Geometry: final body of the model. Coordinates: model frame, mm. Give positions to 0.01 mm unless a question says otherwise; leave off trailing zeros. Write each loop counter-clockwise with the first axis right and the second up, starting at its lowest first coordinate (ties: lowest second). Pieces come first, ordered by that corner, then holes. Notation, with made-up numbers: (71, 10.5) -> (118, 10.5) arc R11 cw to (118, 28.5) -> close; hole circle Ø3 at (35, -28.75). An arc over 180 degrees is marked (long way). Answer as a JSON object with one key per item and string values. Group by question number.
(1) Material intervals for probe 1 along X at (y, z) = (-51.5, 0.2); probe 2 along Y at (x, z) = (15.5, 0.8); probe 3 along Y at (x, z) = (-36, 0.35), sorted ascending.
(2) Section query B-B on y = -46. Output: boundary loops of the cut face in (x, z).
(3) Section query C-C on x = 0. Output: boundary loops of the cut face in (y, z).
(4) Section query A-A on x = 30. Output: boundary loops of the cut face in (y, z), plus the area to 3 significant figures.
(5) Contact query for flat-ended pins moving along their axis: pin 1 Ø0.6 at (x, z) = (63.5, 1) entering from -Y; pin 2 Ø1.1 at (x, z) = (61, 0.5) entering from +Y; pin 3 Ø0.6 at (y, z) = (61.5, 1.5) entering from +X. Output: stop coordinate, or through.
(6) Section query D-D on y = 23. Output: boundary loops of the cut face in (x, z), plus the area to 3 significant figures.
from build123d import *

# Parameters (mm, degrees)
CROQUIS1_W              = 159.22
CROQUIS1_H              = 92
SALIENTE_EXTRUIR1_DEPTH = 2.11
CROQUIS2_R              = 13.6
CORTAR_EXTRUIR1_DEPTH   = 2.11
CROQUIS3_R              = 11
CROQUIS3_R_2            = 1.55
CORTAR_EXTRUIR2_DEPTH   = 2.11
CROQUIS4_W              = 49.61
CROQUIS4_H              = 26
CORTAR_EXTRUIR3_DEPTH   = 2.11
SALIENTE_EXTRUIR2_DEPTH = 2.11
REDONDEO2_R             = 10
CROQUIS5_R              = 8.1
CORTAR_EXTRUIR4_DEPTH   = 2.11
CHAFL_N1_SIZE           = 7
CROQUIS8_R              = 1.7
CORTAR_EXTRUIR5_DEPTH   = 2.11
MATRIZC1_OUTLINE_R      = 1.7
MATRIZC1_DEPTH          = 2.11
CROQUIS9_R              = 1.7
CORTAR_EXTRUIR6_DEPTH   = 2.11
CROQUIS10_R             = 3.75
CORTAR_EXTRUIR7_DEPTH   = 2.11


# Read off the part's stored shape, not the designer's step: MatrizC1
with BuildPart() as part:
    # Croquis1 → Saliente-Extruir1 (new body)
    with BuildSketch(Plane.XY):
        Rectangle(CROQUIS1_W, CROQUIS1_H)
    extrude(amount=SALIENTE_EXTRUIR1_DEPTH)

    # Croquis2 → Cortar-Extruir1 (cut)
    with BuildSketch(Plane.XY.offset(2.11)):
        with Locations((59.61, 0)):
            Circle(CROQUIS2_R)
        with Locations((-59.61, 0)):
            Circle(CROQUIS2_R)
    extrude(amount=-CORTAR_EXTRUIR1_DEPTH, mode=Mode.SUBTRACT)

    # Croquis3 → Cortar-Extruir2 (cut)
    with BuildSketch(Plane.XY.offset(2.11)):
        Circle(CROQUIS3_R)
        with Locations((15.5, 15.5)):
            Circle(CROQUIS3_R_2)
        with Locations((15.5, -15.5)):
            Circle(CROQUIS3_R_2)
        with Locations((-15.5, -15.5)):
            Circle(CROQUIS3_R_2)
        with Locations((-15.5, 15.5)):
            Circle(CROQUIS3_R_2)
    extrude(amount=-CORTAR_EXTRUIR2_DEPTH, mode=Mode.SUBTRACT)

    # Croquis4 → Cortar-Extruir3 (cut)
    with BuildSketch(Plane(origin=(0, 0, 0), x_dir=(-1, 0, 0), z_dir=(0, 0, -1))):
        with Locations((-54.805, 33)):
            Rectangle(CROQUIS4_W, CROQUIS4_H)
        with Locations((-54.805, -33)):
            Rectangle(CROQUIS4_W, CROQUIS4_H)
        with Locations((54.805, -33)):
            Rectangle(CROQUIS4_W, CROQUIS4_H)
        with Locations((54.805, 33)):
            Rectangle(CROQUIS4_W, CROQUIS4_H)
    extrude(amount=-CORTAR_EXTRUIR3_DEPTH, mode=Mode.SUBTRACT)

    # Croquis6 → Saliente-Extruir2 (add)
    with BuildSketch(Plane(origin=(0, 0, 0), x_dir=(-1, 0, 0), z_dir=(0, 0, -1))):
        Polygon((-47, 20), (-30, 20), (-30, 46), (30, 46), (30, 20), (47, 20), (47, 63), (17, 63), (17, 52), (-17, 52), (-17, 63), (-47, 63), align=None)
        Polygon((-30, -46), (30, -46), (30, -20), (47, -20), (47, -63), (17, -63), (17, -52), (-17, -52), (-17, -63), (-47, -63), (-47, -20), (-30, -20), align=None)
    extrude(amount=-SALIENTE_EXTRUIR2_DEPTH)

    # Redondeo2
    redondeo2_edges = [part.edges().sort_by_distance(p)[0] for p in [
        (47, 20, 1.055),
        (47, 63, 1.055),
        (-47, 63, 1.055),
        (-47, 20, 1.055),
        (-47, -20, 1.055),
        (-47, -63, 1.055),
        (47, -63, 1.055),
        (47, -20, 1.055),
        (-79.61, 20, 1.055),
        (-79.61, -20, 1.055),
        (79.61, -20, 1.055),
        (79.61, 20, 1.055),
    ]]
    fillet(redondeo2_edges, radius=REDONDEO2_R)

    # Croquis5 → Cortar-Extruir4 (cut)
    with BuildSketch(Plane(origin=(0, 0, 0), x_dir=(-1, 0, 0), z_dir=(0, 0, -1))):
        with Locations((-30, 46)):
            Circle(CROQUIS5_R)
        with Locations((30, 46)):
            Circle(CROQUIS5_R)
        with Locations((30, -46)):
            Circle(CROQUIS5_R)
        with Locations((-30, -46)):
            Circle(CROQUIS5_R)
        with BuildLine():
            Line((-3.5, -36), (-3.5, -18))
            ThreePointArc((-3.5, -18), (0, -14.5), (3.5, -18))
            Line((3.5, -18), (3.5, -36))
            ThreePointArc((3.5, -36), (0, -39.5), (-3.5, -36))
        make_face()
        with BuildLine():
            Line((-36, 3.5), (-18, 3.5))
            ThreePointArc((-18, 3.5), (-14.5, 0), (-18, -3.5))
            Line((-18, -3.5), (-36, -3.5))
            ThreePointArc((-36, -3.5), (-39.5, 0), (-36, 3.5))
        make_face()
        with BuildLine():
            Line((3.5, 28), (3.5, 18))
            ThreePointArc((3.5, 18), (0, 14.5), (-3.5, 18))
            Line((-3.5, 18), (-3.5, 28))
            ThreePointArc((-3.5, 28), (0, 31.5), (3.5, 28))
        make_face()
        with BuildLine():
            Line((36, -3.5), (18, -3.5))
            ThreePointArc((18, -3.5), (14.5, 0), (18, 3.5))
            Line((18, 3.5), (36, 3.5))
            ThreePointArc((36, 3.5), (39.5, 0), (36, -3.5))
        make_face()
    extrude(amount=-CORTAR_EXTRUIR4_DEPTH, mode=Mode.SUBTRACT)

    # Chaflán1
    chafl_n1_edges = [part.edges().sort_by_distance(p)[0] for p in [
        (17, 52, 1.055),
        (-17, 52, 1.055),
        (-17, -52, 1.055),
        (17, -52, 1.055),
    ]]
    chamfer(chafl_n1_edges, length=CHAFL_N1_SIZE)

    # Croquis8 → Cortar-Extruir5 (cut)
    with BuildSketch(Plane(origin=(0, 0, 0), x_dir=(-1, 0, 0), z_dir=(0, 0, -1))):
        with Locations((-14.722431864, 8.5)):
            Circle(CROQUIS8_R)
    extrude(amount=-CORTAR_EXTRUIR5_DEPTH, mode=Mode.SUBTRACT)

    # MatrizC1 outline → MatrizC1 (cut)
    with BuildSketch(Plane.XY):
        with Locations((-14.722431864, 8.5)):
            Circle(MATRIZC1_OUTLINE_R)
    extrude(amount=MATRIZC1_DEPTH, mode=Mode.SUBTRACT)

    # Croquis9 → Cortar-Extruir6 (cut)
    with BuildSketch(Plane(origin=(0, 0, 0), x_dir=(-1, 0, 0), z_dir=(0, 0, -1))):
        with Locations((-30, 32.5)):
            Circle(CROQUIS9_R)
        with Locations((30, 32.5)):
            Circle(CROQUIS9_R)
        with Locations((-30, 59.5)):
            Circle(CROQUIS9_R)
        with Locations((30, -32.5)):
            Circle(CROQUIS9_R)
        with Locations((-30, -32.5)):
            Circle(CROQUIS9_R)
        with Locations((30, 59.5)):
            Circle(CROQUIS9_R)
    extrude(amount=-CORTAR_EXTRUIR6_DEPTH, mode=Mode.SUBTRACT)

    # Croquis10 → Cortar-Extruir7 (cut)
    with BuildSketch(Plane(origin=(0, 0, 0), x_dir=(-1, 0, 0), z_dir=(0, 0, -1))):
        with Locations((0, 40.6)):
            Circle(CROQUIS10_R)
    extrude(amount=-CORTAR_EXTRUIR7_DEPTH, mode=Mode.SUBTRACT)


solid = part.part
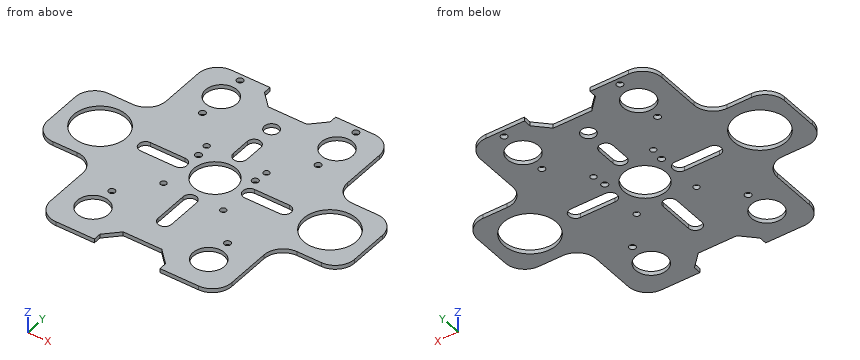
Answer list:
{
 "1": {"probe 1": "-47 to -35.95, -24.05 to 24.05, 35.95 to 47", "probe 2": "-57.5 to -17.05, -13.95 to -2.45, 2.45 to 6.99, 10.01 to 13.95, 17.05 to 57.5", "probe 3": "-63 to -51.44, -40.56 to -3.5, 3.5 to 40.56, 51.44 to 63"},
 "2": {"outline": "(-47, 0) -> (-38.1, 0) -> (-38.1, 2.11) -> (-47, 2.11) -> close; (-21.9, 0) -> (21.9, 0) -> (21.9, 2.11) -> (-21.9, 2.11) -> close; (38.1, 0) -> (47, 0) -> (47, 2.11) -> (38.1, 2.11) -> close"},
 "3": {"outline": "(-52, 0) -> (-39.5, 0) -> (-39.5, 2.11) -> (-52, 2.11) -> close; (-14.5, 0) -> (-11, 0) -> (-11, 2.11) -> (-14.5, 2.11) -> close; (11, 0) -> (14.5, 0) -> (14.5, 2.11) -> (11, 2.11) -> close; (31.5, 0) -> (36.85, 0) -> (36.85, 2.11) -> (31.5, 2.11) -> close; (44.35, 0) -> (52, 0) -> (52, 2.11) -> (44.35, 2.11) -> close"},
 "4": {"outline": "(-63, 0) -> (-54.1, 0) -> (-54.1, 2.11) -> (-63, 2.11) -> close; (-37.9, 0) -> (-34.2, 0) -> (-34.2, 2.11) -> (-37.9, 2.11) -> close; (-30.8, 0) -> (-3.5, 0) -> (-3.5, 2.11) -> (-30.8, 2.11) -> close; (3.5, 0) -> (30.8, 0) -> (30.8, 2.11) -> (3.5, 2.11) -> close; (34.2, 0) -> (37.9, 0) -> (37.9, 2.11) -> (34.2, 2.11) -> close; (54.1, 0) -> (57.8, 0) -> (57.8, 2.11) -> (54.1, 2.11) -> close; (61.2, 0) -> (63, 0) -> (63, 2.11) -> (61.2, 2.11) -> close", "area": "161 mm2"},
 "5": {"pin 1": "y = -20", "pin 2": "y = 20", "pin 3": "x = 42.72"},
 "6": {"outline": "(-49.86, 0) -> (-3.5, 0) -> (-3.5, 2.11) -> (-49.86, 2.11) -> close; (3.5, 0) -> (49.86, 0) -> (49.86, 2.11) -> (3.5, 2.11) -> close", "area": "196 mm2"}
}
